The listing builds one solid part. Answer for the finished solid, in the listing's coordinates (mm). Face numbers are marked on the shaded views. A direction names the side the tool comes from. Give positions to 0.01 mm unless a question says otherwise; leave off trailing zeros. Order: outer loops, then holes, each group sorted by start corner. A loop starts at its lowest first (then second) coordinate and runs counter-clockwise, first axis right, second up. Notation, with made-up numbers: (-31, 62) -> (-20, 62) arc R23 ccw to (-20, 74) -> close; hole circle Ø11 at (44.25, 85). An arc over 180 degrees is marked (long way). Answer as a JSON object with one key per item and string values. Group by question number.
```python
from build123d import *
from build123d.topology import SkipClean

# Parameters (mm, degrees)
SKETCH1_W           = 70
SKETCH1_H           = 70
BOSS_EXTRUDE1_DEPTH = 20
SKETCH3_W           = 10
SKETCH3_H           = 70
BOSS_EXTRUDE2_DEPTH = 50
SKETCH4_R           = 25
SKETCH4_R_2         = 20.325
BOSS_EXTRUDE3_DEPTH = 20
FILLET1_R           = 10
SKETCH5_W           = 20.15
SKETCH5_H           = 40.15
CUT_EXTRUDE1_DEPTH  = 5
CUT_EXTRUDE3_DEPTH  = 140
CUT_EXTRUDE4_DEPTH  = 2.5
SKETCH9_W           = 50
SKETCH9_H           = 70
CUT_EXTRUDE5_DEPTH  = 5
SKETCH8_4_R         = 6.6
SKETCH8_4_R_2       = 3.1
CUT_EXTRUDE8_DEPTH  = 6
SKETCH12_R          = 2.25
CUT_EXTRUDE9_DEPTH  = 8
SKETCH12_3_W        = 1.2
SKETCH12_3_H        = 7.15
CUT_EXTRUDE10_DEPTH = 1.6
SKETCH8_5_R         = 3.1
CUT_EXTRUDE11_DEPTH = 10
SKETCH13_R          = 10.525
CUT_EXTRUDE12_DEPTH = 10
FILLET2_R           = 5


with BuildPart() as part:
    # Sketch1 → Boss-Extrude1 (new body)
    with BuildSketch(Plane(origin=(0, 0, 0), x_dir=(1, 0, 0), z_dir=(0, 1, 0))):
        Rectangle(SKETCH1_W, SKETCH1_H)
    extrude(amount=BOSS_EXTRUDE1_DEPTH)

    # Sketch3 → Boss-Extrude2 (add)
    with BuildSketch(Plane(origin=(0, 20, 0), x_dir=(1, 0, 0), z_dir=(0, 1, 0))):
        with Locations((-30, 0)):
            Rectangle(SKETCH3_W, SKETCH3_H)
        with Locations((30, 0)):
            Rectangle(SKETCH3_W, SKETCH3_H)
    extrude(amount=BOSS_EXTRUDE2_DEPTH)

    # Sketch4 → Boss-Extrude3 (add)
    with BuildSketch(Plane(origin=(0, -20, 0), x_dir=(-1, 0, 0), z_dir=(0, -1, 0))):
        with Locations(Location((0, 0, 0), (0, 0, 90))):
            Circle(SKETCH4_R)
        with Locations(Location((0, 0, 0), (0, 0, 90))):
            Circle(SKETCH4_R_2, mode=Mode.SUBTRACT)
    extrude(amount=-BOSS_EXTRUDE3_DEPTH)

    # Fillet1
    fillet1_edges = [part.edges().sort_by_distance(p)[0] for p in [
        (0, 0, 25),
    ]]
    fillet(fillet1_edges, radius=FILLET1_R - 0.0001)  # a hair under: the kernel refuses the full size

    # Sketch5 → Cut-Extrude1 (cut)
    with BuildSketch(Plane(origin=(35, 0, 0), x_dir=(0, 0, -1), z_dir=(1, 0, 0))):
        with Locations((0, 38.075)):
            Rectangle(SKETCH5_W, SKETCH5_H)
    extrude(amount=-CUT_EXTRUDE1_DEPTH, mode=Mode.SUBTRACT)

    # Sketch6 → Cut-Extrude3 (cut)
    with BuildSketch(Plane(origin=(35, 0, 0), x_dir=(0, 0, -1), z_dir=(1, 0, 0))):
        with BuildLine():
            Line((-35, 70), (-35, 20))
            add(Edge.make_bspline(
                [(-35, 20), (-31.043970013, 56.876347524), (-23.178818695, 69.774444442), (-1.193819381, 70)],
                knots=[0, 0, 0, 0, 0.690984823, 0.690984823, 0.690984823, 0.690984823], degree=3))
            Line((-1.193819381, 70), (-35, 70))
        make_face()
        with BuildLine():
            add(Edge.make_bspline(
                [(35, 20), (31.043970013, 56.876347524), (23.178818695, 69.774444442), (1.193819381, 70)],
                knots=[0, 0, 0, 0, 0.690984823, 0.690984823, 0.690984823, 0.690984823], degree=3))
            Line((35, 20), (35, 70))
            Line((35, 70), (1.193819381, 70))
        make_face()
    extrude(amount=-CUT_EXTRUDE3_DEPTH, mode=Mode.SUBTRACT)

    # Sketch8 → Cut-Extrude4 (cut)
    with BuildSketch(Plane(origin=(30, 0, 0), x_dir=(0, 0, -1), z_dir=(1, 0, 0))):
        with BuildLine():
            ThreePointArc((10.075, 48.075), (7.124100826, 55.199100815), (1.7e-08, 58.15))
            ThreePointArc((1.7e-08, 58.15), (-7.124100815, 55.199100826), (-10.075, 48.075))
            ThreePointArc((-10.075, 48.075), (-9.828227841, 45.858795474), (-9.1, 43.751156224))
            Line((-9.1, 43.751156224), (-9.1, 48.075))
            Line((-9.1, 48.075), (-6.6, 48.075))
            ThreePointArc((-6.6, 48.075), (0, 54.675), (6.6, 48.075))
            Line((6.6, 48.075), (9.1, 48.075))
            Line((9.1, 48.075), (9.1, 43.751156224))
            ThreePointArc((9.1, 43.751156224), (9.828227841, 45.858795474), (10.075, 48.075))
        make_face()
        with BuildLine():
            Line((-9.1, 48.075), (-9.1, 43.751156224))
            ThreePointArc((-9.1, 43.751156224), (0, 38), (9.1, 43.751156224))
            Line((9.1, 43.751156224), (9.1, 48.075))
            Line((9.1, 48.075), (6.6, 48.075))
            ThreePointArc((6.6, 48.075), (0, 41.475), (-6.6, 48.075))
            Line((-6.6, 48.075), (-9.1, 48.075))
        make_face()
        with BuildLine():
            ThreePointArc((9.1, 43.751156224), (0, 38), (-9.1, 43.751156224))
            Line((-9.1, 43.751156224), (-9.1, 23.375))
            Line((-9.1, 23.375), (9.1, 23.375))
            Line((9.1, 23.375), (9.1, 43.751156224))
        make_face()
        with BuildLine():
            ThreePointArc((6.6, 48.075), (0, 54.675), (-6.6, 48.075))
            Line((-6.6, 48.075), (-3.1, 48.075))
            ThreePointArc((-3.1, 48.075), (0, 51.175), (3.1, 48.075))
            Line((3.1, 48.075), (6.6, 48.075))
        make_face()
        with BuildLine():
            Line((-3.1, 48.075), (-6.6, 48.075))
            ThreePointArc((-6.6, 48.075), (0, 41.475), (6.6, 48.075))
            Line((6.6, 48.075), (3.1, 48.075))
            ThreePointArc((3.1, 48.075), (0, 44.975), (-3.1, 48.075))
        make_face()
    extrude(amount=-CUT_EXTRUDE4_DEPTH, mode=Mode.SUBTRACT)

    # Sketch9 → Cut-Extrude5 (cut)
    with BuildSketch(Plane(origin=(0, 20, 0), x_dir=(1, 0, 0), z_dir=(0, 1, 0))):
        Rectangle(SKETCH9_W, SKETCH9_H)
    extrude(amount=-CUT_EXTRUDE5_DEPTH, mode=Mode.SUBTRACT)

    # Sketch8<4> → Cut-Extrude8 (cut)
    with SkipClean():  # the faces are left unmerged after this step: merging them gives an invalid solid
        with BuildSketch(Plane(origin=(30, 0, 0), x_dir=(0, 0, -1), z_dir=(1, 0, 0))):
            with Locations((0, 48.075)):
                Circle(SKETCH8_4_R)
            with Locations((0, 48.075)):
                Circle(SKETCH8_4_R_2, mode=Mode.SUBTRACT)
        extrude(amount=-CUT_EXTRUDE8_DEPTH, mode=Mode.SUBTRACT)


with BuildPart() as cut_extrude8_piece_1:
    # of the separate pieces the step leaves, piece 1, a body of its own (cut_extrude8_pieces)
    add(part.part.solids().sort_by_distance((0, 0, -34.9999))[0])

    # Sketch12 → Cut-Extrude9 (cut)
    with BuildSketch(Plane(origin=(35, 0, 0), x_dir=(0, 0, -1), z_dir=(1, 0, 0))):
        with Locations((-5.005, 63.05)):
            Circle(SKETCH12_R)
        with Locations((5.005, 63.05)):
            Circle(SKETCH12_R)
    extrude(amount=-CUT_EXTRUDE9_DEPTH, mode=Mode.SUBTRACT)

    # Sketch12<3> → Cut-Extrude10 (cut)
    with BuildSketch(Plane(origin=(35, 0, 0), x_dir=(0, 0, -1), z_dir=(1, 0, 0))):
        with Locations((0, 61.725)):
            Rectangle(SKETCH12_3_W, SKETCH12_3_H)
    extrude(amount=-CUT_EXTRUDE10_DEPTH, mode=Mode.SUBTRACT)

    # Sketch13 → Cut-Extrude12 (cut)
    with BuildSketch(Plane.ZY.offset(35)):
        with Locations((0, 48.075)):
            Circle(SKETCH13_R)
    extrude(amount=-CUT_EXTRUDE12_DEPTH, mode=Mode.SUBTRACT)

    # Fillet2
    fillet2_edges = [cut_extrude8_piece_1.edges().sort_by_distance(p)[0] for p in [
        (-35, 10, 35),
        (35, 10, 35),
        (35, 10, -35),
        (-35, 10, -35),
    ]]
    fillet(fillet2_edges, radius=FILLET2_R)


with BuildPart() as cut_extrude8_piece_2:
    # of the separate pieces the step leaves, piece 2, a body of its own (cut_extrude8_pieces)
    add(part.part.solids().sort_by_distance((25, 48.075, -3.1))[0])

    # Sketch8<5> → Cut-Extrude11 (cut)
    with BuildSketch(Plane(origin=(30, 0, 0), x_dir=(0, 0, -1), z_dir=(1, 0, 0))):
        with Locations((0, 48.075)):
            Circle(SKETCH8_5_R)
    extrude(amount=-CUT_EXTRUDE11_DEPTH, mode=Mode.SUBTRACT)


solid = cut_extrude8_piece_1.part
```
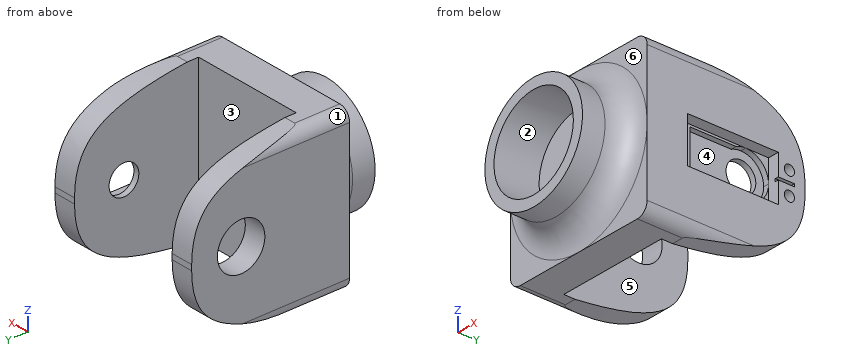
(1) Which of the six approach directions +Z, -Z, +X, -X, +Y, -Y give full straight-line access (tool end or side, diameter ignored) to the marked faces 4, 5 and 6?
(2) A cutting plane is placed at B-B (y = 50). State how many separate pieces and enclosed holes the cut face has, and give its area (3 significant figures).
(3) Find the intervals of material crossed by line 1 along X through (y, z) = (63, 14); line 2 along X through (y, z) = (35.5, 0.5); line 3 along Z through (x, y) = (30, 63), in increasing order. Write a range as [from, to].
(4) For a pull along Z with two mould halves and no side action, classify the marked faces 1, 2 and 3 as +Z half, -Z half, draft (parallel to the pull), parting line (faces both ways), or undercut.
(5) Flat-ended cylindrical pins translate along their axes: pin 1 Ø0.8 at (x, y) = (34.5, 63) entering from -Z; pin 2 Ø2.5 at (x, y) = (32, 46) entering from +Z; pin 3 Ø0.8 at (x, z) = (28.5, -3.5) entering from +Y; pin 4 Ø22 at (y, z) = (37.5, 0) entering from +X. Find the tip coordinate at first contact, or state that the pin passes through.
(6) A cutting plane is placed at A-A (y = -13). Determine the outline of the cut face in (x, z) (3 decimals).
Check sheet entries:
{
 "1": {"face 4": "+X", "face 5": "+Z, -Z, +Y", "face 6": "-Y"},
 "2": {"separate pieces": "4", "enclosed holes": "0", "area": "776 mm2"},
 "3": {"line 1": "x = [-35, -25], [25, 35]", "line 2": "x = [-35, -25], [25, 27.5]", "line 3": "z = [-21.37, -7.25], [-2.76, 2.76], [7.25, 21.37]"},
 "4": {"face 1": "+Z half", "face 2": "undercut", "face 3": "draft"},
 "5": {"pin 1": "stops at z = -21.77", "pin 2": "stops at z = 30.77", "pin 3": "stops at y = 69.95", "pin 4": "stops at x = 35"},
 "6": {"outline": "circle Ø50 at (0, 0); hole circle Ø40.65 at (0, 0)"}
}
